Study the drawing (mm; zero at the part's minimum x, y, z) and answer. Give positions to 0.01 mm unless a question says otherwise; leave off trailing zeros. Write each loop counter-clockwise with the first axis right and the second up, starting at its lowest first coordinate (ties: lowest second). Pieces come first, ordered by that corner, then holes. Notation, with made-up numbers: (9.5, 34) - (62.5, 34) arc R22 ccw to (62.5, 46) - close; hole circle Ø4 at (-19.5, -4). An arc over 180 degrees is marked (long way). Return JSON: item names as keys, results as strings.
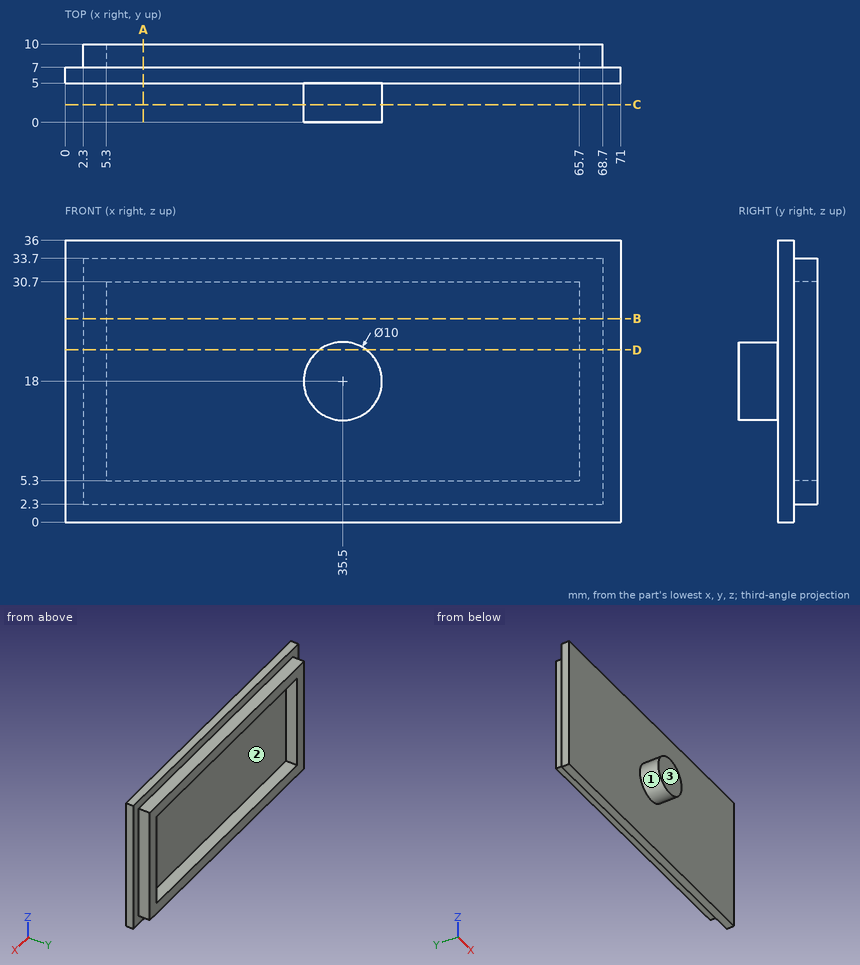
Item 1: A cutting plane is placed at B-B on z = 26. Determine the outline of the cut face in (x, y).
Answer below:
{"outline": "(0, 5) - (71, 5) - (71, 7) - (68.7, 7) - (68.7, 10) - (65.7, 10) - (65.7, 7) - (5.3, 7) - (5.3, 10) - (2.3, 10) - (2.3, 7) - (0, 7) - close"}
Item 2: The mould has two halves that part along X. Classify the marked faces 1, 2 and 3: +X half, -X half, draft (parallel to the pull), parting line (faces both ways), or undercut.
Answer below:
{"face 1": "parting line", "face 2": "undercut", "face 3": "draft"}
Item 3: A cutting plane is placed at C-C on y = 2.25. Determine the outline of the cut face in (x, z), then the cut area to 3 significant figures.
Answer below:
{"outline": "circle Ø10 at (35.5, 18)", "area": "78.5 mm²"}
Item 4: Consider L1, parallel to Z at x = 56.5, y = 7.5; L2, parallel to X at y = 7.75, z = 11; L3, parallel to Y at x = 9, z = 16. Determine where each line is inside the solid, lowest interval first.
Answer below:
{"L1": "z = 2.3 to 5.3, 30.7 to 33.7", "L2": "x = 2.3 to 5.3, 65.7 to 68.7", "L3": "y = 5 to 7"}
Item 5: A cutting plane is placed at D-D on z = 22. Determine the outline of the cut face in (x, y).
Answer below:
{"outline": "(0, 5) - (32.5, 5) - (32.5, 0) - (38.5, 0) - (38.5, 5) - (71, 5) - (71, 7) - (68.7, 7) - (68.7, 10) - (65.7, 10) - (65.7, 7) - (5.3, 7) - (5.3, 10) - (2.3, 10) - (2.3, 7) - (0, 7) - close"}
Item 6: Flat-ended cylindrical pins translate along their axes: P1, Ø2, axis at y = 8.5, z = 32.5, coming from the +X side; P2, Ø3.5, axis at x = 48, y = 9, coming from the -Z side; P3, Ø1.5, axis at y = 9, z = 22.5, coming from the -X side; P4, Ø3, axis at y = 2.5, z = 5.5, coming from the -X side. Find the tip coordinate at first contact, or state that the pin passes through.
Answer below:
{"P1": "stops at x = 68.7", "P2": "stops at z = 2.3", "P3": "stops at x = 2.3", "P4": "passes through"}
Item 7: A cutting plane is placed at A-A on x = 10. Determine the outline of the cut face in (y, z), then the cut area to 3 significant figures.
Answer below:
{"outline": "(5, 0) - (7, 0) - (7, 2.3) - (10, 2.3) - (10, 5.3) - (7, 5.3) - (7, 30.7) - (10, 30.7) - (10, 33.7) - (7, 33.7) - (7, 36) - (5, 36) - close", "area": "90.0 mm²"}
